The listing builds one solid part. Answer for the finished solid, in the listing's coordinates (mm). Give positions to 0.01 mm unless a question says otherwise; leave off trailing zeros. Write each loop counter-clockwise with the first axis right and the second up, starting at its lowest first coordinate (ties: lowest second). Pieces come first, ordered by that corner, then holes. Notation, with made-up numbers: M 7.25,16.25 L 21.25,16.25 A33 ccw 21.25,51.25 Z; hole C 53.5,56.25 d6. An arc over 180 degrees is marked long. Return JSON: item names as keys, results as strings.
from build123d import *

# Parameters (mm, degrees)
SKETCH1_R           = 54.656342245
SKETCH1_R_2         = 1.7
SKETCH1_R_3         = 3
BOSS_EXTRUDE1_DEPTH = 1


with BuildPart() as part:
    # Sketch1 → Boss-Extrude1 (new body)
    with BuildSketch(Plane.XY):
        Circle(SKETCH1_R)
        with Locations((0, 35)):
            Circle(SKETCH1_R_2, mode=Mode.SUBTRACT)
        with Locations((30.310889132, -17.5)):
            Circle(SKETCH1_R_2, mode=Mode.SUBTRACT)
        with Locations((-30.310889132, -17.5)):
            Circle(SKETCH1_R_2, mode=Mode.SUBTRACT)
        with Locations((0, 10)):
            Circle(SKETCH1_R_3, mode=Mode.SUBTRACT)
        with Locations((8.660254038, 5)):
            Circle(SKETCH1_R_3, mode=Mode.SUBTRACT)
        with Locations((8.660254038, -5)):
            Circle(SKETCH1_R_3, mode=Mode.SUBTRACT)
        with Locations((0, -10)):
            Circle(SKETCH1_R_3, mode=Mode.SUBTRACT)
        with Locations((-8.660254038, -5)):
            Circle(SKETCH1_R_3, mode=Mode.SUBTRACT)
        with Locations((-8.660254038, 5)):
            Circle(SKETCH1_R_3, mode=Mode.SUBTRACT)
    extrude(amount=BOSS_EXTRUDE1_DEPTH)


solid = part.part
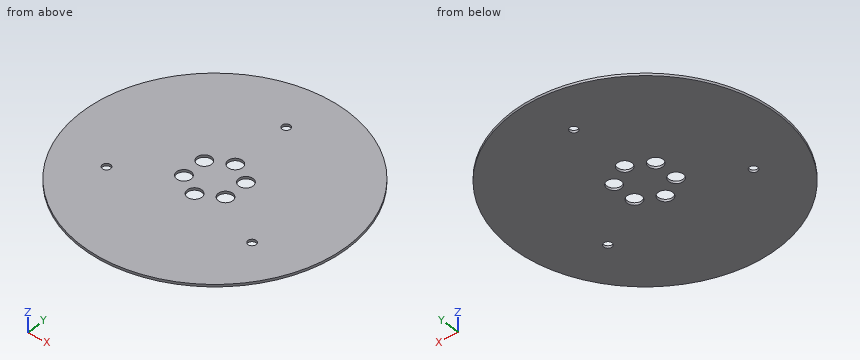
Item 1: A cutting plane is placed at D-D, the plane y = -5. Write down the section's boundary in (x, z), plus the area to 3 significant figures.
Geometry results:
{"outline": "M -54.43,0 L -11.66,0 L -11.66,1 L -54.43,1 Z; M -5.66,0 L 5.66,0 L 5.66,1 L -5.66,1 Z; M 11.66,0 L 54.43,0 L 54.43,1 L 11.66,1 Z", "area": "96.9 mm2"}
Item 2: A cutting plane is placed at C-C, the plane y = 35. Write down the section's boundary in (x, z).
Geometry results:
{"outline": "M -41.98,0 L -1.7,0 L -1.7,1 L -41.98,1 Z; M 1.7,0 L 41.98,0 L 41.98,1 L 1.7,1 Z"}
Item 3: Find the intervals of material crossed by line 1 (Y direction, x = 0, z = 0.55); line 2 (Y direction, x = -30, z = 0.55); line 3 (X direction, y = 40, z = 0.9), in increasing order.
Geometry results:
{"line 1": "y = -54.66 to -13, -7 to 7, 13 to 33.3, 36.7 to 54.66", "line 2": "y = -45.69 to -19.17, -15.83 to 45.69", "line 3": "x = -37.25 to 37.25"}
Item 4: A cutting plane is placed at A-A, the plane x = 0. Write down the section's boundary in (y, z), plus the area to 3 significant figures.
Geometry results:
{"outline": "M -54.66,0 L -13,0 L -13,1 L -54.66,1 Z; M -7,0 L 7,0 L 7,1 L -7,1 Z; M 13,0 L 33.3,0 L 33.3,1 L 13,1 Z; M 36.7,0 L 54.66,0 L 54.66,1 L 36.7,1 Z", "area": "93.9 mm2"}
Item 5: A cutting plane is placed at B-B, the plane z = 0.55. Count the separate pieces of the cut face and the enclosed holes in it, plus the area to 3 significant figures.
Geometry results:
{"separate pieces": "1", "enclosed holes": "9", "area": "9,190 mm2"}
